Check sheet for the modelled part. Datum: model origin and axes. Units: mm. A direction names the side the tool comes from. Round coordinates to 2 decimals unless told otherwise and drop trailing zeros. Return JSON: item names as keys, results as strings.
from build123d import *

# Parameters (mm, degrees)
SKETCH_1_R      = 3.4
SKETCH_1_R_2    = 2.95
EXTRUDE_1_DEPTH = 600


with BuildPart() as part:
    # 草图1 → 凸台-拉伸1 (new body)
    with BuildSketch(Plane.XY):
        Polygon((-5.378679656, -7.5), (5.378679656, -7.5), (10.05, -12.171320344), (10.05, -17.2), (4.15, -17.2), (4.15, -20), (20, -20), (20, -4.15), (17.2, -4.15), (17.2, -10.05), (12.171320344, -10.05), (7.5, -5.378679656), (7.5, 5.378679656), (12.171320344, 10.05), (17.2, 10.05), (17.2, 4.15), (20, 4.15), (20, 20), (4.15, 20), (4.15, 17.2), (10.05, 17.2), (10.05, 12.171320344), (5.378679656, 7.5), (-5.378679656, 7.5), (-10.05, 12.171320344), (-10.05, 17.2), (-4.15, 17.2), (-4.15, 20), (-20, 20), (-20, 4.15), (-17.2, 4.15), (-17.2, 10.05), (-12.171320344, 10.05), (-7.5, 5.378679656), (-7.5, -5.378679656), (-12.171320344, -10.05), (-17.2, -10.05), (-17.2, -4.15), (-20, -4.15), (-20, -20), (-4.15, -20), (-4.15, -17.2), (-10.05, -17.2), (-10.05, -12.171320344), align=None)
        Circle(SKETCH_1_R, mode=Mode.SUBTRACT)
        with Locations((15.025, 15.025)):
            Circle(SKETCH_1_R_2, mode=Mode.SUBTRACT)
        with Locations(Location((-15.025, 15.025, 0), (0, 0, 180))):
            Circle(SKETCH_1_R_2, mode=Mode.SUBTRACT)
        with Locations((-15.025, -15.025)):
            Circle(SKETCH_1_R_2, mode=Mode.SUBTRACT)
        with Locations(Location((15.025, -15.025, 0), (0, 0, 180))):
            Circle(SKETCH_1_R_2, mode=Mode.SUBTRACT)
    extrude(amount=EXTRUDE_1_DEPTH)


solid = part.part
Q1. Scan lines: probe 1 along X at (y, z) = (-5, 369.5); probe 2 along Y at (x, z) = (-13, 446); probe 3 along X at (y, z) = (16.5, 485.5). Record each from-to range of solid material in increasing order. Write a range as [from, to].
Answer key:
{"probe 1": "x = [-20, -17.2], [-7.5, 7.5], [17.2, 20]", "probe 2": "y = [-20, -17.17], [-12.88, -10.05], [10.05, 12.88], [17.17, 20]", "probe 3": "x = [-20, -17.58], [-12.47, -10.05], [10.05, 12.47], [17.58, 20]"}
Q2. Sectioned sample at A-A (z = 108). State how many separate pieces and enclosed holes the cut face has, plus the area to 3 significant figures.
Answer key:
{"separate pieces": "1", "enclosed holes": "5", "area": "669 mm²"}
Q3. Draft check along Y on faces 1 (the face through (20, 12, 296)), 2 (the face through (-12, 20, 296)), 3 (the face through (-7.5, 0, 296)). Enter one of: released by +Y, released by -Y, zero draft, split by the parting line, or undercut.
Answer key:
{"face 1": "zero draft", "face 2": "released by +Y", "face 3": "undercut"}
Q4. Depth check by flat-ended pin: P1, Ø5.5, axis at x = 0, z = 302.5, coming from the +Y side; P2, Ø3, axis at y = 1.5, z = 360, coming from the -X side. Enter the tip coordinate at first touch or a pass-through.
Answer key:
{"P1": "stops at y = 7.5", "P2": "stops at x = -7.5"}
Q5. Tool access check on faces 4 (the face through (20, -12, 296)), 5 (the face through (0, -7.5, 296)). Record the directions out of +Z, -Z, +X, -X, +Y, -Y that give a thin tool (end or side, any length) a straight path to the whole face; none if there is none.
Answer key:
{"face 4": "+Z, -Z, +X, +Y, -Y", "face 5": "+Z, -Z"}
